from build123d import *

# Parameters (mm, degrees)
SALIENTE_EXTRUIR1_DEPTH = 7.5
CROQUIS2_R              = 3
CORTAR_EXTRUIR1_DEPTH   = 170.871274794


with BuildPart() as part:
    # Croquis1 → Saliente-Extruir1 (new, symmetric)
    with BuildSketch(Plane.XY):
        with BuildLine():
            Line((12.330243842, 32.118869601), (21.650635095, 37.5))
            ThreePointArc((21.650635095, 37.5), (21.650635095, 12.5), (0, 0))
            Line((0, 0), (-165, 0))
            Line((-165, 0), (-165, 15))
            Line((-165, 15), (0, 15))
            ThreePointArc((0, 15), (10.548585327, 20.402148489), (12.330243842, 32.118869601))
        make_face()
    extrude(amount=SALIENTE_EXTRUIR1_DEPTH, both=True)

    # Croquis2 → Cortar-Extruir1 (cut, through all)
    with BuildSketch(Plane.XY.offset(7.5)):
        with Locations((-120, 7.5)):
            Circle(CROQUIS2_R)
    extrude(amount=-CORTAR_EXTRUIR1_DEPTH, mode=Mode.SUBTRACT)


solid = part.part
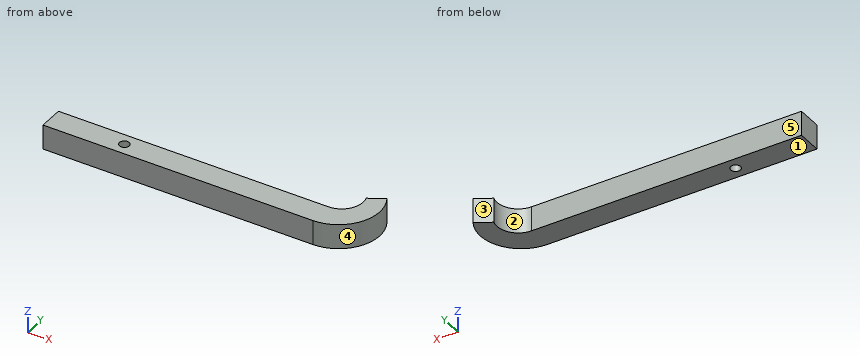
Check sheet for the modelled part. Datum: model origin and axes. Units: mm. Face numbers are marked on the shaded views. A direction names the side the tool comes from. Round coordinates to 2 decimals unless told otherwise and drop trailing zeros. Write each loop counter-clockwise with the first axis right and the second up, starting at its lowest first coordinate (ties: lowest second). Pieces come first, ordered by that corner, then holes. Notation, with made-up numbers: (62.25, 81.5) - (102.25, 81.5) arc R23 cw to (102.25, 110.5) - close; hole circle Ø2 at (18.25, -38.75). An arc over 180 degrees is marked (long way). Return JSON: item names as keys, results as strings.
Q1. Cross-section at C-C (y = 7.5). Record the boundary of the cut face in (x, z), then the cut area to 3 significant figures.
Returned:
{"outline": "(-165, -7.5) - (-123, -7.5) - (-123, 7.5) - (-165, 7.5) - close; (-117, -7.5) - (17.85, -7.5) - (17.85, 7.5) - (-117, 7.5) - close", "area": "2,650 mm²"}
Q2. Scan lines: L1, parallel to Y at x = -120, z = -1.25; L2, parallel to Y at x = -24.5, z = 5.75; L3, parallel to X at y = 6, z = 4.75. Record each from-to range of solid material in increasing order. Write a range as from..to.
Returned:
{"L1": "y = 0..4.5, 10.5..15", "L2": "y = 0..15", "L3": "x = -165..-122.6, -117.4..16.25"}
Q3. Cross-section at B-B (z = 3.75). Record the boundary of the cut face in (x, y).
Returned:
{"outline": "(-165, 0) - (0, 0) arc R25 ccw to (21.65, 37.5) - (12.33, 32.12) arc R13 cw to (0, 15) - (-165, 15) - close; hole circle Ø6 at (-120, 7.5)"}
Q4. Cross-section at A-A (x = -120). Record the boundary of the cut face in (y, z).
Returned:
{"outline": "(0, -7.5) - (4.5, -7.5) - (4.5, 7.5) - (0, 7.5) - close; (10.5, -7.5) - (15, -7.5) - (15, 7.5) - (10.5, 7.5) - close"}
Q5. Access from +Z, -Z, +X, -X, +Y, -Y to the whole of each face (thin tool, end or side, straight path). Record for the marked faces 4 and 5.
Returned:
{"face 4": "+Z, -Z, +X", "face 5": "+Z, -Z, -X, +Y"}
Q6. Draft check along Y on the marked faces 1, 2 and 3. Enter one of: released by +Y, released by -Y, zero draft, split by the parting line, or undercut.
Returned:
{"face 1": "zero draft", "face 2": "undercut", "face 3": "released by +Y"}
Q7. Cross-section at D-D (y = 26.5). Record the boundary of the cut face in (x, z).
Returned:
{"outline": "(12.91, -7.5) - (24.95, -7.5) - (24.95, 7.5) - (12.91, 7.5) - close"}
Q8. Depth check by flat-ended pin: P1, Ø8, axis at x = -4.5, z = 1, coming from the +Y side; P2, Ø6, axis at x = 5, z = -1.5, coming from the +Y side; P3, Ø4, axis at y = 25.5, z = 5.5, coming from the +X side. Enter the tip coordinate at first touch or a pass-through.
Returned:
{"P1": "stops at y = 15", "P2": "stops at y = 17.75", "P3": "stops at x = 25"}
